Autodesk Inventor part; units mm, degrees
ref_plane "YZ Plane" through (0, 0, 0) normal (1, 0, 0) x (0, 1, 0)
ref_plane "XZ Plane" through (0, 0, 0) normal (0, 1, 0) x (-1, 0, 0)
ref_plane "XY Plane" through (0, 0, 0) normal (0, 0, 1) x (1, 0, 0)
sketch "Sketch1" plane through (0, 0, 0) normal (0, 0, 1) x (1, 0, 0)
  line L0 (0, 0) -> (-12, 0)
  line L1 (-12, 0) -> (-12, 10)
  line L2 (-12, 10) -> (0, 10)
  line L3 (0, 10) -> (0, 0)
  dimension "d0" = 12
  dimension "d1" = 10
extrude "Extrusion1" add sketch "Sketch1" along normal blind 27.9
sketch "Sketch2" plane through (0, 0, 0) normal (0, 0, -1) x (-1, 0, 0)
  circle A0 centre (6, 5) radius 2
  line L0 (12, 0) -> (0, 0)
  line L1 (0, 0) -> (0, 10)
  point P0 (6, 0)
  dimension "d4" = 5
  dimension "d5" = 6
  dimension "d9" = 4
extrude "Extrusion2" add sketch "Sketch2" along normal blind 0.7
sketch "Sketch5" plane through (-6, 5, -0.7) normal (0, 0, -1) x (-1, 0, 0)
  circle A0 centre (0, 0) radius 2
  arc A1 (-1.118, 1) -> (1.118, 1) centre (0, 0) ccw
  line L0 (-1.118, 1) -> (1.118, 1)
  point P0 (-6, -5)
  point P1 (0.4397, 1)
  dimension "d14" = 3
  dimension "d15" = 1
extrude "Extrusion4" add sketch "Sketch5" along normal blind 9.3 contours L0 A1
fillet "Fillet1" radius 2 4 edges at (-12, 10, 13.95) (0, 10, 13.95) (-12, 0, 13.95) (0, 0, 13.95)
properties part number "motor"
Geometry check sheet. Reference: the model listing, model coordinates, mm. A direction names the side the tool comes from. Give positions to 0.01 mm unless a question says otherwise; leave off trailing zeros. Order: outer loops, then holes, each group sorted by start corner. A loop starts at its lowest first (then second) coordinate and runs counter-clockwise, first axis right, second up. Notation, with made-up numbers: (46, 14.25) - (52, 14.25) arc R25 cw to (52, 53.25) - close; hole circle Ø10 at (15.5, 75). An arc over 180 degrees is marked (long way). Answer as a JSON object with one key per item and string values.
(1) Material ranges on line 1 (Z direction, x = -11, y = 4.5); line 2 (Z direction, x = -5.25, y = 6.5); line 3 (X direction, y = 9.5, z = 9), recorded low to high.
Report:
{"line 1": "0 to 27.9", "line 2": "-0.7 to 27.9", "line 3": "-11.32 to -0.68"}
(2) Cross-section at C-C (x = -6). Record the cut outline in (y, z), then the cut area to 3 significant figures.
Report:
{"outline": "(0, 0) - (3, 0) - (3, -0.7) - (3.5, -0.7) - (3.5, -10) - (6, -10) - (6, -0.7) - (7, -0.7) - (7, 0) - (10, 0) - (10, 27.9) - (0, 27.9) - close", "area": "305 mm^2"}
(3) Tool access check on faces 1 (the flat face through (-6, 6, -5)), 2 (the flat face through (-6.1, 2.8, 0)), 3 (the cylindrical face through (-11.43, 0.6, 14.15)). Record the directions out of +Z, -Z, +X, -X, +Y, -Y that give a thin tool (end or side, any length) a straight path to the whole face; none if there is none.
Report:
{"face 1": "-Z, +X, -X, +Y", "face 2": "-Z", "face 3": "+Z, -Z, -X, -Y"}
(4) Cross-section at B-B (y = 5). Record the cut outline in (x, z), then the cut area to 4 significant figures.
Report:
{"outline": "(-12, 0) - (-8, 0) - (-8, -0.7) - (-7.5, -0.7) - (-7.5, -10) - (-4.5, -10) - (-4.5, -0.7) - (-4, -0.7) - (-4, 0) - (0, 0) - (0, 27.9) - (-12, 27.9) - close", "area": "365.5 mm^2"}
(5) Cross-section at D-D (x = -2.75). Record the cut outline in (y, z), then the cut area to 3 significant figures.
Report:
{"outline": "(0, 0) - (10, 0) - (10, 27.9) - (0, 27.9) - close", "area": "279 mm^2"}
(6) Draft check along Y on faces 4 (the cylindrical face through (-0.57, 9.4, 14.15)), 5 (the cylindrical face through (-4.4, 6.2, -0.3)), 6 (the flat face through (-6, 6.4, -0.7)). Enter one of: released by +Y, released by -Y, zero draft, split by the parting line, or undercut.
Report:
{"face 4": "released by +Y", "face 5": "split by the parting line", "face 6": "zero draft"}
(7) Depth check by flat-ended pin: pin 1 Ø4 at (x, y) = (-2.5, 1) entering from -Z; pin 2 Ø1.8 at (x, z) = (-5.5, -6.5) entering from +Y; pin 3 Ø2 at (y, z) = (4, -6) entering from -X. Enter the tip coordinate at first touch or a pass-through.
Report:
{"pin 1": "z = 0", "pin 2": "y = 6", "pin 3": "x = -7.5"}
(8) Cross-section at A-A (z = 0.5). Record the cut outline in (x, y).
Report:
{"outline": "(-12, 2) arc R2 ccw to (-10, 0) - (-2, 0) arc R2 ccw to (0, 2) - (0, 8) arc R2 ccw to (-2, 10) - (-10, 10) arc R2 ccw to (-12, 8) - close"}
